from build123d import *

# Parameters (mm, degrees)
SKETCH_3_W          = 1.5
SKETCH_3_H          = 12
CUT_EXTRUDE_1_DEPTH = 1


with BuildPart() as part:
    # 草图2 → 旋转1 (revolve)
    with BuildSketch(Plane(origin=(0, 0, 0), x_dir=(0, 0, -1), z_dir=(1, 0, 0))):
        Polygon((0, 0), (0, 6), (3, 6), (3, 4), (19, 4), (19, 3), (26, 3), (26, 0), align=None)
    revolve(axis=Axis((0, 0, 0), (0, 0, -1)))

    # 草图3 → 切除-拉伸1 (cut)
    with BuildSketch(Plane.XY):
        Rectangle(SKETCH_3_W, SKETCH_3_H)
    extrude(amount=-CUT_EXTRUDE_1_DEPTH, mode=Mode.SUBTRACT)


solid = part.part
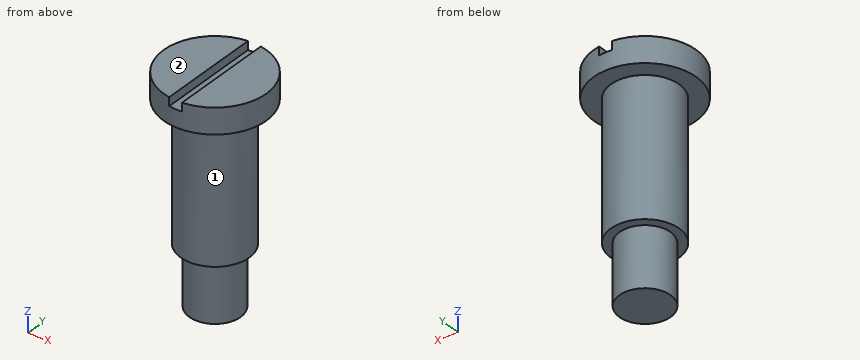
Input: part model. Units: mm. Frame: model coordinates. Face numbers are marked on the shaded views. A direction names the side the tool comes from. Give positions to 0.01 mm unless a question says otherwise; leave off trailing zeros. Write each loop counter-clockwise with the first axis right and the second up, starting at its lowest first coordinate (ties: lowest second). Pieces come first, ordered by that corner, then holes.
Q1. Section D-D, the plane y = -1.25. Output: boundary loops of the cut face in (x, z), plus the area to 3 significant figures.
Q2. Section C-C, the plane z = -24.5. Output: boundary loops of the cut face in (x, y).
Q3. First-contact query: P1, Ø1.5, axis at x = 2.5, z = -18.5, coming from the +Y side; P2, Ø4, axis at y = -1.5, z = -13.5, coming from the +X side; P3, Ø1.1, axis at y = 2.5, z = -0.5, coming from the -X side. Flat tips, straight axial feed; report the tip coordinate or a pass-through.
Q4. Set-up query: the marked faces 1 and 2. Return all of +Z, -Z, +X, -X, +Y, -Y with unobstructed straight access to the full face (end or side cutting, diameter ignored); none if empty.
Q5. Material intervals for probe 1 along Z at (x, y) = (-1.5, 3.5); probe 2 along Z at (x, y) = (4.75, 1); probe 3 along X at (y, z) = (-3.25, -9), sorted ascending.
Q6. Section B-B, the plane y = 0. Output: boundary loops of the cut face in (x, z).
Q7. Section A-A, the plane x = 0. Output: boundary loops of the cut face in (y, z).
Filled in:
1. outline: (-5.87, -3) - (-3.8, -3) - (-3.8, -19) - (-2.73, -19) - (-2.73, -26) - (2.73, -26) - (2.73, -19) - (3.8, -19) - (3.8, -3) - (5.87, -3) - (5.87, 0) - (0.75, 0) - (0.75, -1) - (-0.75, -1) - (-0.75, 0) - (-5.87, 0) - close
1. area: 193 mm2
2. outline: circle Ø6 at (0, 0)
3. P1: stops at y = 3.6
3. P2: stops at x = 4
3. P3: stops at x = -5.67
4. face 1: -Z
4. face 2: +Z, +X, -X, +Y, -Y
5. probe 1: z = -19 to 0
5. probe 2: z = -3 to 0
5. probe 3: x = -2.33 to 2.33
6. outline: (-6, -3) - (-4, -3) - (-4, -19) - (-3, -19) - (-3, -26) - (3, -26) - (3, -19) - (4, -19) - (4, -3) - (6, -3) - (6, 0) - (0.75, 0) - (0.75, -1) - (-0.75, -1) - (-0.75, 0) - (-6, 0) - close
7. outline: (-6, -3) - (-4, -3) - (-4, -19) - (-3, -19) - (-3, -26) - (3, -26) - (3, -19) - (4, -19) - (4, -3) - (6, -3) - (6, -1) - (-6, -1) - close
